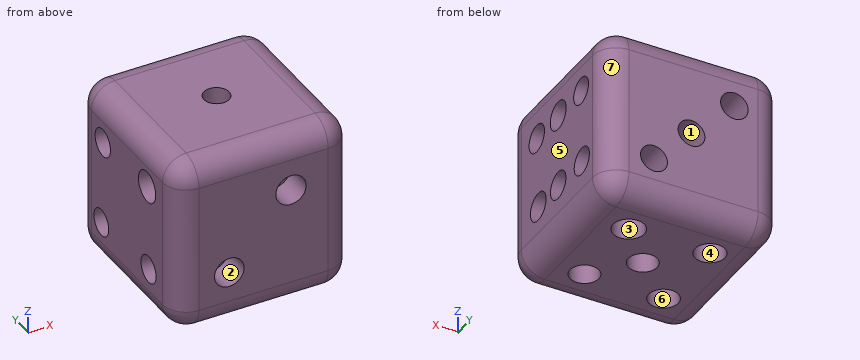
```python
from build123d import *

# Parameters (mm, degrees)
F0_W      = 38.1
F0_H      = 38.1
F1_DEPTH  = 38.1
F2_R      = 5.08
F3_R      = 2.734829
F4_DEPTH  = 6.35
F5_R      = 3.201955
F5_R_2    = 3.279746
F6_DEPTH  = 6.35
F7_R      = 3.135653
F7_R_2    = 3.122225
F7_R_3    = 3.201953
F7_R_4    = 3.241083
F7_R_5    = 3.393092
F8_DEPTH  = 6.35
F9_R      = 2.898913
F9_R_2    = 2.984612
F9_R_3    = 2.913371
F10_DEPTH = 6.35
F11_R     = 3.026556
F11_R_2   = 2.956325
F11_R_3   = 3.380686
F11_R_4   = 2.913369
F12_DEPTH = 25.4
F13_R     = 3.026552
F13_R_2   = 3.122223
F13_R_3   = 3.026557
F13_R_4   = 3.081587
F13_R_5   = 2.984611
F13_R_6   = 2.913373
F14_DEPTH = 6.35


with BuildPart() as f1:
    # F0 (on Front) → F1 (new body)
    with BuildSketch(Plane.XZ):
        with Locations((-0.434836, -16.367298)):
            Rectangle(F0_W, F0_H)
    extrude(amount=F1_DEPTH)

    # F2
    f2_edges = [f1.edges().sort_by_distance(p)[0] for p in [
        (-19.484836, -19.05, 2.682702),
        (-0.434836, -38.1, 2.682702),
        (18.615164, -19.05, 2.682702),
        (-0.434836, 0, 2.682702),
        (18.615164, 0, -16.367298),
        (18.615164, -19.05, -35.417298),
        (-0.434836, 0, -35.417298),
        (18.615164, -38.1, -16.367298),
        (-19.484836, -38.1, -16.367298),
        (-0.434836, -38.1, -35.417298),
        (-19.484836, -19.05, -35.417298),
        (-19.484836, 0, -16.367298),
    ]]
    fillet(f2_edges, radius=F2_R)

    # F3 (on face) → F4 (cut)
    with BuildSketch(Plane.XY.offset(2.682702)):
        with Locations((0, -18.842936)):
            Circle(F3_R)
    extrude(amount=-F4_DEPTH, mode=Mode.SUBTRACT)

    # F5 (on face) → F6 (cut)
    with BuildSketch(Plane.XZ.offset(38.1)):
        with Locations((-7.827066, -23.771087)):
            Circle(F5_R)
        with Locations((5.507934, -9.276522)):
            Circle(F5_R_2)
    extrude(amount=-F6_DEPTH, mode=Mode.SUBTRACT)

    # F7 (on face) → F8 (cut)
    with BuildSketch(Plane(origin=(0, 0, -35.417298), x_dir=(1, 0, 0), z_dir=(0, 0, -1))):
        with Locations((0, 19.132826)):
            Circle(F7_R)
        with Locations((7.827064, 27.829565)):
            Circle(F7_R_2)
        with Locations((-9.27652, 27.829565)):
            Circle(F7_R_3)
        with Locations((-9.566413, 10.146196)):
            Circle(F7_R_4)
        with Locations((7.827064, 10.436087)):
            Circle(F7_R_5)
    extrude(amount=-F8_DEPTH, mode=Mode.SUBTRACT)

    # F9 (on face) → F10 (cut)
    with BuildSketch(Plane(origin=(0, 0, 0), x_dir=(-1, 0, 0), z_dir=(0, 1, 0))):
        with Locations((0, -17.103586)):
            Circle(F9_R)
        with Locations((9.27652, -7.827065)):
            Circle(F9_R_2)
        with Locations((-8.116957, -25.510436)):
            Circle(F9_R_3)
    extrude(amount=-F10_DEPTH, mode=Mode.SUBTRACT)

    # F11 (on face) → F12 (cut)
    with BuildSketch(Plane(origin=(-19.484836, 0, 0), x_dir=(0, -1, 0), z_dir=(-1, 0, 0))):
        with Locations((9.566412, -7.247283)):
            Circle(F11_R)
        with Locations((27.539674, -25.510436)):
            Circle(F11_R_2)
        with Locations((26.959889, -6.957392)):
            Circle(F11_R_3)
        with Locations((8.986631, -25.800327)):
            Circle(F11_R_4)
    extrude(amount=-F12_DEPTH, mode=Mode.SUBTRACT)

    # F13 (on face) → F14 (cut)
    with BuildSketch(Plane.YZ.offset(18.615164)):
        with Locations((-18.553045, -24.060978)):
            Circle(F13_R)
        with Locations((-18.553045, -8.116957)):
            Circle(F13_R_2)
        with Locations((-26.959889, -8.406848)):
            Circle(F13_R_3)
        with Locations((-26.380109, -24.350869)):
            Circle(F13_R_4)
        with Locations((-9.276524, -24.060978)):
            Circle(F13_R_5)
        with Locations((-9.566412, -7.827065)):
            Circle(F13_R_6)
    extrude(amount=-F14_DEPTH, mode=Mode.SUBTRACT)


solid = f1.part
```
The listing builds one solid part. Answer for the finished solid, in the listing's coordinates (mm). Face numbers are marked on the shaded views. A direction names the side the tool comes from. Coordinates: 2 decimals unless noted, no trailing zeros. Write each loop counter-clockwise with the first axis right and the second up, starting at its lowest first coordinate (ties: lowest second). Pieces come first, ordered by that corner, then holes. Notation, with made-up numbers: M -34,82.25 L 6,82.25 A17 cw 6,91.25 Z; hole C 21,19 d10. An arc over 180 degrees is marked long. Use a Markdown table: item, result. Add a question column.
1. Given P1, Ø11, axis at x = 7.83, y = -10.44, coming from the -Z side; P2, Ø1.9, axis at x = 0, y = -20, coming from the -Z side; P3, Ø1.9, axis at x = -9.5, z = -25, coming from the -Y side; P4, Ø1.8, axis at y = -27.5, z = -24.5, coming from the -X side, each flat-ended and moving along its own axis, determine where each tip first touches the part or whether it passes through.
2. Section C-C (x = 0) is taken. Give the vertices of the cut face in (y, z).
3. Section A-A (y = -4) is taken. Give the vertices of the cut face in (x, z), plus the area to 3 significant figures.
4. Straight lines are drawn through the part: line 1 along Y through (x, z) = (-15, -27.5); line 2 along Z through (x, y) = (-14.5, -11.5); line 3 along Z through (x, y) = (-8.5, -8.5). For each, find the intervals that lie inside material, in ascending order. Write a range as [from, to].
5. For a pull along Y with two mould halves and no side action, classify the marked faces 4, 5, 6 and 7 as +Y half, -Y half, draft (parallel to the pull), parting line (faces both ways), or undercut.
6. Section D-D (y = -18) is taken. Give the vertices of the cut face in (x, z), plus the area to 3 significant figures.
7. Section B-B (z = -3) is taken. Give the vertices of the cut face in (x, y), plus the area to 3 significant figures.
8. Which of the six approach directions +Z, -Z, +X, -X, +Y, -Y give full straight-line access (tool end or side, diameter ignored) to the marked faces 1, 2 and 3?
Data:
| question | item | result |
|---|---|---|
| 1 | P1 | stops at z = -35.42 |
| 1 | P2 | stops at z = -29.07 |
| 1 | P3 | stops at y = -31.75 |
| 1 | P4 | stops at x = 5.92 |
| 2 | outline | M -38.1,-30.34 A5.08 ccw -33.02,-35.42 L -22.27,-35.42 L -22.27,-29.07 L -16,-29.07 L -16,-35.42 L -5.08,-35.42 A5.08 ccw 0,-30.34 L 0,-20 L -6.35,-20 L -6.35,-14.2 L 0,-14.2 L 0,-2.4 A5.08 ccw -5.08,2.68 L -16.11,2.68 L -16.11,-3.67 L -21.58,-3.67 L -21.58,2.68 L -33.02,2.68 A5.08 ccw -38.1,-2.4 Z; hole C -27.54,-25.51 d5.91; hole C -26.96,-6.96 d6.76; hole C -9.57,-7.25 d6.05; hole C -8.99,-25.8 d5.83 |
| 3 | outline | M -19.37,-30.34 A4.96 ccw -14.4,-35.3 L 13.54,-35.3 A4.96 ccw 18.5,-30.34 L 18.5,-2.4 A4.96 ccw 13.54,2.57 L -14.4,2.57 A4.96 ccw -19.37,-2.4 Z; hole C -9.28,-7.83 d5.97; hole C 0,-17.1 d5.8; hole C 8.12,-25.51 d5.83 |
| 3 | area | 1,330 mm2 |
| 4 | line 1 | y = [-38.07, -29.73], [-25.35, -11.35], [-6.62, -0.03] |
| 4 | line 2 | z = [-35.42, -27.27], [-24.33, -9.58], [-4.92, 2.68] |
| 4 | line 3 | z = [-29.07, -28.67], [-22.93, -10.08], [-4.41, 2.68] |
| 5 | face 4 | undercut |
| 5 | face 5 | draft |
| 5 | face 6 | undercut |
| 5 | face 7 | +Y half |
| 6 | outline | M -19.48,-30.34 A5.08 ccw -14.4,-35.42 L -2.92,-35.42 L -2.92,-29.07 L 2.92,-29.07 L 2.92,-35.42 L 13.54,-35.42 A5.08 ccw 18.62,-30.34 L 18.62,-27.04 L 12.27,-27.04 L 12.27,-21.09 L 18.62,-21.09 L 18.62,-11.19 L 12.27,-11.19 L 12.27,-5.04 L 18.62,-5.04 L 18.62,-2.4 A5.08 ccw 13.54,2.68 L 2.6,2.68 L 2.6,-3.67 L -2.6,-3.67 L -2.6,2.68 L -14.4,2.68 A5.08 ccw -19.48,-2.4 Z |
| 6 | area | 1,280 mm2 |
| 7 | outline | M -19.48,-33.02 A5.08 ccw -14.4,-38.1 L 13.54,-38.1 A5.08 ccw 18.62,-33.02 L 18.62,-5.08 A5.08 ccw 13.54,0 L -14.4,0 A5.08 ccw -19.48,-5.08 Z; hole C 0,-18.84 d5.47 |
| 7 | area | 1,410 mm2 |
| 8 | face 1 | +Y |
| 8 | face 2 | -Y |
| 8 | face 3 | -Z |
